Part model, mm, in its own coordinate system. Coordinates: 2 decimals unless noted, no trailing zeros. Order: outer loops, then holes, each group sorted by start corner. A loop starts at its lowest first (then second) coordinate and runs counter-clockwise, first axis right, second up.
1) Cut at A-A (x = 50.8). List the corners of the cut face in (y, z).
2) Wall check: L1, parallel to X at y = 0.3, z = 0.5; L2, parallel to X at y = 1.45, z = 18; L3, parallel to X at y = 1.5, z = 3. Give the ranges that are in metal, low to high.
3) Pin check, flat tips, straight feed: pin 1 Ø7 at (x, z) = (0, 25.4) entering from +Y; pin 2 Ø0.5 at (x, y) = (26.5, 1) entering from -Z; pin 3 Ø3.5 at (x, z) = (50.8, 25.4) entering from -Y; pin 4 Ø0.5 at (y, z) = (0.5, 7) entering from -X. Stop position of each tip, or through.
4) Cut at B-B (z = 7). List the corners of the cut face in (x, y), and give its area (3 significant figures).
5) Cut at D-D (x = 0). List the corners of the cut face in (y, z), and give its area (3 significant figures).
6) Cut at C-C (y = 0.3). Give the number of separate pieces and of enclosed holes in the cut face, and give its area (3 significant figures).
Autodesk Inventor part; units mm, degrees
ref_plane "YZ Plane" through (0, 0, 0) normal (1, 0, 0) x (0, 1, 0)
ref_plane "XZ Plane" through (0, 0, 0) normal (0, 1, 0) x (-1, 0, 0)
ref_plane "XY Plane" through (0, 0, 0) normal (0, 0, 1) x (1, 0, 0)
sketch "main" plane through (0, 0, 0) normal (0, 0, 1) x (1, 0, 0)
  circle A0 centre (9.0037, 34.4943) radius 2.1844
  line L0 (21.7037, 28.1443) -> (9.0037, 15.4443)
  line L1 (34.4037, 28.1443) -> (21.7037, 28.1443)
  circle A1 centre (34.4037, 34.4943) radius 2.1844
  arc A2 (34.4037, 28.1443) -> (34.4037, 40.8443) centre (34.4037, 34.4943) ccw
  arc A3 (-17.5684, -13.257) -> (-15.6972, -14.455) centre (-14.1357, -9.9557) ccw
  circle A4 centre (-14.1357, -9.9557) radius 2.0828
  line L2 (-15.6972, -14.455) -> (6.9217, -22.3047)
  circle A5 centre (-14.1255, 15.4443) radius 2.0828
  line L3 (-29.4913, -0.8595) -> (-17.5684, -13.257)
  arc A6 (-29.6904, 5.5225) -> (-29.4913, -0.8595) centre (-26.0586, 2.4417) ccw
  line L4 (-0.6786, 39.7231) -> (-29.6904, 5.5225)
  line L5 (9.0037, -3.6057) -> (9.0037, 15.4443)
  line L6 (15.3537, -9.9557) -> (34.4037, -9.9557)
  line L7 (15.3537, -9.9557) -> (9.0037, -3.6057)
  circle A7 centre (34.4037, -16.3057) radius 2.1844
  arc A8 (34.4037, -22.6557) -> (34.4037, -9.9557) centre (34.4037, -16.3057) ccw
  circle A9 centre (9.0037, -16.3057) radius 2.1844
  arc A10 (6.9217, -22.3047) -> (9.0037, -22.6557) centre (9.0037, -16.3057) ccw
  line L8 (9.0037, -22.6557) -> (34.4037, -22.6557)
  arc A11 (0.516, 40.5978) -> (-0.6786, 39.7231) centre (1.7426, 37.6693) ccw
  arc A12 (9.1983, 44.0073) -> (8.3903, 43.896) centre (9.0036, 42.4318) ccw
  line L9 (0.516, 40.5978) -> (8.3903, 43.896)
  line L10 (35.1824, 40.7963) -> (9.1983, 44.0073)
  point P0 (6.3419, 6.6617)
  point P1 (9.0037, 28.1443)
  point P2 (0.2724, 40.8443)
  point P3 (-32.4736, 2.2415)
  point P4 (9.0037, -9.9557)
  dimension "d0" = 4.1656
  dimension "d1" = 9.525
  dimension "d2" = 12.7
  dimension "d3" = 12.7
  dimension "d4" = 6.35
  dimension "d5" = 6.35
  dimension "d6" = 4.1656
  dimension "d7" = 4.7625
  dimension "d9" = 3.175
  dimension "d12" = 48.5394
  dimension "d14" = 3.175
  dimension "d16" = 25.4
  dimension "d17" = 48.5291
  dimension "d18" = 6.35
sketch "Sketch1" plane through (0, 0, 0) normal (0, 1, 0) x (-1, 0, 0)
  circle A0 centre (0.0003, 25.4) radius 2.1844
  line L0 (-6.3499, 12.7001) -> (-19.0497, 25.4002)
  line L1 (-6.35, 0.0001) -> (-6.3499, 12.7001)
  circle A1 centre (0, 0) radius 2.1844
  arc A2 (-6.35, 0.0001) -> (6.35, -0.0001) centre (0, 0) ccw
  arc A3 (-47.7507, 51.9726) -> (-48.9487, 50.1014) centre (-44.4495, 48.5399) ccw
  circle A4 centre (-44.4495, 48.5399) radius 2.0828
  line L2 (-48.9487, 50.1014) -> (-56.7987, 27.4825)
  circle A5 centre (-19.0495, 48.5293) radius 2.0828
  line L3 (-35.3531, 63.8953) -> (-47.7507, 51.9726)
  arc A6 (-28.9711, 64.0944) -> (-35.3531, 63.8953) centre (-32.0519, 60.4626) ccw
  line L4 (5.2292, 35.0822) -> (-28.9711, 64.0944)
  line L5 (-38.0997, 25.4004) -> (-19.0497, 25.4002)
  line L6 (-44.4498, 19.0505) -> (-44.45, 0.0005)
  line L7 (-44.4498, 19.0505) -> (-38.0997, 25.4004)
  circle A7 centre (-50.8, 0.0005) radius 2.1844
  arc A8 (-57.15, 0.0006) -> (-44.45, 0.0005) centre (-50.8, 0.0005) ccw
  circle A9 centre (-50.7997, 25.4005) radius 2.1844
  arc A10 (-56.7987, 27.4825) -> (-57.1497, 25.4006) centre (-50.7997, 25.4005) ccw
  line L8 (-57.1497, 25.4006) -> (-57.15, 0.0006)
  arc A11 (6.1038, 33.8876) -> (5.2292, 35.0822) centre (3.1753, 32.661) ccw
  arc A12 (9.5133, 25.2052) -> (9.402, 26.0132) centre (7.9378, 25.3999) ccw
  line L9 (6.1038, 33.8876) -> (9.402, 26.0132)
  line L10 (6.3021, -0.7788) -> (9.5133, 25.2052)
  point P0 (0, 0)
extrude "Extrusion1" add sketch "Sketch1" along normal blind 1.5875
properties part number "gusset" material "Acetal Resin, White"
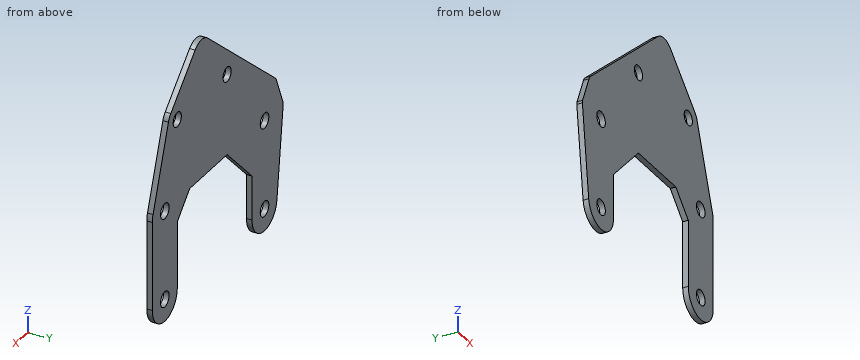
Geometry check:
1. outline: (0, -6.35) - (1.59, -6.35) - (1.59, -2.18) - (0, -2.18) - close; (0, 2.18) - (1.59, 2.18) - (1.59, 23.22) - (0, 23.22) - close; (0, 27.58) - (1.59, 27.58) - (1.59, 44.77) - (0, 44.77) - close
2. L1: x = -6.46 to -2.13, 2.13 to 6.35, 44.45 to 48.67, 52.93 to 57.15
2. L2: x = -8.62 to 11.65, 44.45 to 57.15
2. L3: x = -6.77 to 6.35, 44.45 to 57.15
3. pin 1: stops at y = 1.59
3. pin 2: stops at z = 25.4
3. pin 3: passes through
3. pin 4: stops at x = -7.29
4. outline: (-7.26, 0) - (6.35, 0) - (6.35, 1.59) - (-7.26, 1.59) - close; (44.45, 0) - (57.15, 0) - (57.15, 1.59) - (44.45, 1.59) - close
4. area: 41.8 mm2
5. outline: (0, -6.35) - (1.59, -6.35) - (1.59, -2.18) - (0, -2.18) - close; (0, 2.18) - (1.59, 2.18) - (1.59, 23.22) - (0, 23.22) - close; (0, 27.58) - (1.59, 27.58) - (1.59, 39.52) - (0, 39.52) - close
5. area: 58.9 mm2
6. separate pieces: 1
6. enclosed holes: 6
6. area: 2,470 mm2
